Part model, mm, in its own coordinate system. Face numbers are marked on the shaded views. A direction names the side the tool comes from. Round coordinates to 2 decimals unless told otherwise and drop trailing zeros. Order: outer loops, then holes, each group sorted by start corner. A loop starts at its lowest first (then second) coordinate and runs counter-clockwise, first axis right, second up. Notation, with made-up numbers: M 55.25,77.5 L 108.25,77.5 A23 cw 108.25,101.5 Z; hole C 23,-12 d4. An arc over 180 degrees is marked long. One line per question, with ' | ' between items.
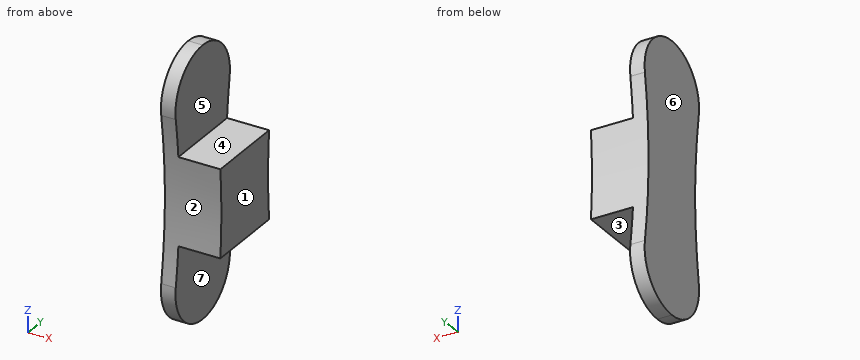
from build123d import *

# Parameters (mm, degrees)
BOSS_EXTRUDE1_DEPTH     = 35
CUT_EXTRUDE1_DEPTH      = 146.0965196
CUT_EXTRUDE1_DEPTH_BACK = 146.0965196
SKETCH4_W               = 52
SKETCH4_H               = 56


with BuildPart() as part:
    # Sketch1 → Boss-Extrude1 (new body)
    with BuildSketch(Plane(origin=(0, 0, 0), x_dir=(0, 0, -1), z_dir=(1, 0, 0))):
        with BuildLine():
            ThreePointArc((-4.051298915, 27.705360079), (-21.182969216, 18.310702204), (-28, 0))
            Line((-28, 0), (28, 0))
            ThreePointArc((28, 0), (18.310702204, 21.182969216), (-4.051298915, 27.705360079))
        make_face()
        with BuildLine():
            Line((28, 0), (-28, 0))
            ThreePointArc((-28, 0), (-21.182969216, -18.310702204), (-4.051298915, -27.705360079))
            ThreePointArc((-4.051298915, -27.705360079), (18.310702204, -21.182969216), (28, 0))
        make_face()
        with BuildLine():
            ThreePointArc((-105.948701085, 27.705360079), (-88.817030784, 18.310702204), (-82, 0))
            Line((-82, 0), (-28, 0))
            ThreePointArc((-28, 0), (-21.182969216, 18.310702204), (-4.051298915, 27.705360079))
            ThreePointArc((-4.051298915, 27.705360079), (-55, 24), (-105.948701085, 27.705360079))
        make_face()
        with BuildLine():
            Line((-28, 0), (-82, 0))
            ThreePointArc((-82, 0), (-88.817030784, -18.310702204), (-105.948701085, -27.705360079))
            ThreePointArc((-105.948701085, -27.705360079), (-55, -24), (-4.051298915, -27.705360079))
            ThreePointArc((-4.051298915, -27.705360079), (-21.182969216, -18.310702204), (-28, 0))
        make_face()
        with BuildLine():
            ThreePointArc((-105.948701085, 27.705360079), (-128.310702204, 21.182969216), (-138, 0))
            Line((-138, 0), (-82, 0))
            ThreePointArc((-82, 0), (-88.817030784, 18.310702204), (-105.948701085, 27.705360079))
        make_face()
        with BuildLine():
            Line((-82, 0), (-138, 0))
            ThreePointArc((-138, 0), (-128.310702204, -21.182969216), (-105.948701085, -27.705360079))
            ThreePointArc((-105.948701085, -27.705360079), (-88.817030784, -18.310702204), (-82, 0))
        make_face()
    extrude(amount=BOSS_EXTRUDE1_DEPTH)

    # Sketch4 → Cut-Extrude1 (cut, two sides: drawn at the far end of the back side and taken through both)
    with BuildSketch(Plane(origin=(0, 0, 0), x_dir=(1, 0, 0), z_dir=(0, 1, 0)).offset(-CUT_EXTRUDE1_DEPTH_BACK)):
        with Locations((35, 0)):
            Rectangle(SKETCH4_W, SKETCH4_H)
        with Locations((35, -110)):
            Rectangle(SKETCH4_W, SKETCH4_H)
    extrude(amount=CUT_EXTRUDE1_DEPTH + CUT_EXTRUDE1_DEPTH_BACK, mode=Mode.SUBTRACT)


solid = part.part
1) Drop flat-ended pins along their axis: pin 1 (8 mm diameter, centred on x = 28, y = 1.5, fed in from +Z); pin 2 (3 mm diameter, centred on y = -11, z = 24.5, fed in from -X); pin 3 (12 mm diameter, centred on x = 14.5, y = -10.5, fed in from +Z); pin 4 (4 mm diameter, centred on y = -9, z = 5, fed in from +X). Give the stop position or say it passes through.
The answers:
pin 1: stops at z = 82 | pin 2: stops at x = 0 | pin 3: stops at z = 136.8 | pin 4: stops at x = 9
2) Saw through at D-D (x = 23.5). List the corners of the cut face in (y, z) (3 decimals), plus the area to 3 significant figures.
The answers:
outline: M -25.037,28 L 25.037,28 A352.125 cw 25.037,82 L -25.037,82 A352.125 cw Z | area: 2,630 mm²
3) Saw through at A-A (x = 2). List the corners of the cut face in (y, z) (3 decimals).
The answers:
outline: M -27.705,4.051 A28 ccw long 27.705,4.051 A352.125 cw 27.705,105.949 A28 ccw long -27.705,105.949 A352.125 cw Z
4) Saw through at B-B (y = 4.5). List the corners of the cut face in (x, z), plus the area to 3 significant figures.
The answers:
outline: M 0,-27.64 L 9,-27.64 L 9,28 L 35,28 L 35,82 L 9,82 L 9,137.64 L 0,137.64 Z | area: 2,890 mm²
5) Two-plate mould, pull along Z, no slides. Class the marked faces 1, 2, 3 and 4: released by +Z, released by -Z, zero draft, split by the parting line, or undercut.
The answers:
face 1: zero draft | face 2: undercut | face 3: released by -Z | face 4: released by +Z
6) Which spindle directions (+Z, -Z, +X, -X, +Y, -Y) get a long thin tool onto all of the face, cutting with end or side? Do the marked faces 5, 6 and 7. Say none if no direction does.
The answers:
face 5: +Z, +X, +Y, -Y | face 6: +Z, -Z, -X, +Y, -Y | face 7: -Z, +X, +Y, -Y
7) Saw through at C-C (z = 26.5). List the corners of the cut face in (x, y), plus the area to 3 significant figures.
The answers:
outline: M 0,-25.16 L 9,-25.16 L 9,25.16 L 0,25.16 Z | area: 453 mm²
8) Probe line 1 (Z direction, x = 15.5, y = 3.5); line 2 (X direction, y = -4, z = -0.5); line 3 (Y direction, x = 2, z = 110.5). List the from-to ranges inside material, lowest first. Write a range as [from, to].
The answers:
line 1: z = [28, 82] | line 2: x = [0, 9] | line 3: y = [-28, 28]
